```python
from build123d import *

# Parameters (mm, degrees)
SKETCH_2_W                       = 41
SKETCH_2_H                       = 41
EXTRUDE_1_DEPTH                  = 14.3
EXTRUDE_2_DEPTH                  = 1
SKETCH_4_R                       = 7.75
EXTRUDE_3_DEPTH                  = 8
SKETCH_5_R                       = 5.5
EXTRUDE_4_DEPTH                  = 2
SKETCH_6_R                       = 7
EXTRUDE_5_DEPTH                  = 5.2
FILLET_1_R                       = 1
EXTRUDE_6_DEPTH                  = 0.4
SKETCH_11_W                      = 11.5
SKETCH_11_H                      = 6
CUT_EXTRUDE_1_DEPTH              = 7
SKETCH_12_W                      = 11
SKETCH_12_H                      = 4.8
EXTRUDE_7_DEPTH                  = 8.5
SKETCH_13_R                      = 0.5
EXTRUDE_8_DEPTH                  = 3
SKETCH_14_R                      = 1
EXTRUDE_9_DEPTH                  = 2
EXTRUDE_9_DIRECTION_2_REACH      = 48.597
EXTRUDE_9_DIRECTION_2_END_RADIUS = 7.75
SKETCH_15_R                      = 1.5
EXTRUDE_10_DEPTH                 = 1.5


with BuildPart() as part:
    # 草图2 → 凸台-拉伸1 (new body)
    with BuildSketch(Plane.XY):
        Rectangle(SKETCH_2_W, SKETCH_2_H)
    extrude(amount=EXTRUDE_1_DEPTH)

    # 草图3 → 凸台-拉伸2 (add)
    with BuildSketch(Plane.XY.offset(14.3)):
        with BuildLine():
            Line((-11.808683246, 15.061374439), (-6.531779188, 9.784470381))
            ThreePointArc((-6.531779188, 9.784470381), (-5.963517237, 9.501263014), (-5.339283039, 9.617279066))
            ThreePointArc((-5.339283039, 9.617279066), (0, 11), (5.339283039, 9.617279066))
            ThreePointArc((5.339283039, 9.617279066), (5.963517237, 9.501263014), (6.531779188, 9.784470381))
            Line((6.531779188, 9.784470381), (11.808683246, 15.061374439))
            ThreePointArc((11.808683246, 15.061374439), (15.061374439, 15.061374439), (15.061374439, 11.808683246))
            Line((15.061374439, 11.808683246), (9.784470381, 6.531779188))
            ThreePointArc((9.784470381, 6.531779188), (9.501263014, 5.963517237), (9.617279066, 5.339283039))
            ThreePointArc((9.617279066, 5.339283039), (11, 0), (9.617279066, -5.339283039))
            ThreePointArc((9.617279066, -5.339283039), (9.501263014, -5.963517237), (9.784470381, -6.531779188))
            Line((9.784470381, -6.531779188), (15.061374439, -11.808683246))
            ThreePointArc((15.061374439, -11.808683246), (15.061374439, -15.061374439), (11.808683246, -15.061374439))
            Line((11.808683246, -15.061374439), (6.531779188, -9.784470381))
            ThreePointArc((6.531779188, -9.784470381), (5.963517237, -9.501263014), (5.339283039, -9.617279066))
            ThreePointArc((5.339283039, -9.617279066), (0, -11), (-5.339283039, -9.617279066))
            ThreePointArc((-5.339283039, -9.617279066), (-5.963517237, -9.501263014), (-6.531779188, -9.784470381))
            Line((-6.531779188, -9.784470381), (-11.808683246, -15.061374439))
            ThreePointArc((-11.808683246, -15.061374439), (-15.061374439, -15.061374439), (-15.061374439, -11.808683246))
            Line((-15.061374439, -11.808683246), (-9.784470381, -6.531779188))
            ThreePointArc((-9.784470381, -6.531779188), (-9.501263014, -5.963517237), (-9.617279066, -5.339283039))
            ThreePointArc((-9.617279066, -5.339283039), (-11, 0), (-9.617279066, 5.339283039))
            ThreePointArc((-9.617279066, 5.339283039), (-9.501263014, 5.963517237), (-9.784470381, 6.531779188))
            Line((-9.784470381, 6.531779188), (-15.061374439, 11.808683246))
            ThreePointArc((-15.061374439, 11.808683246), (-15.061374439, 15.061374439), (-11.808683246, 15.061374439))
        make_face()
    extrude(amount=EXTRUDE_2_DEPTH)

    # 草图4 → 凸台-拉伸3 (add)
    with BuildSketch(Plane.XY.offset(15.3)):
        Circle(SKETCH_4_R)
    extrude(amount=EXTRUDE_3_DEPTH)

    # 草图5 → 凸台-拉伸4 (add)
    with BuildSketch(Plane.XY.offset(23.3)):
        Circle(SKETCH_5_R)
    extrude(amount=EXTRUDE_4_DEPTH)

    # 草图6 → 凸台-拉伸5 (add)
    with BuildSketch(Plane.XY.offset(25.3)):
        Circle(SKETCH_6_R)
    extrude(amount=EXTRUDE_5_DEPTH)

    # 草图7 → 切除-旋转3 (revolve, cut)
    with BuildSketch(Plane(origin=(0, 0, 0), x_dir=(1, 0, 0), z_dir=(0, 1, 0)), mode=Mode.PRIVATE) as cut_revolve_3_sk:
        with BuildLine():
            Line((-6.8, -30.5), (-5.688128428, -28.574181946))
            ThreePointArc((-5.688128428, -28.574181946), (-4.965242644, -28.084479441), (-4.133231164, -28.349298811))
            ThreePointArc((-4.133231164, -28.349298811), (-2.225332237, -29.572063929), (0, -30))
            Line((0, -30), (0, -30.5))
            Line((0, -30.5), (-6.8, -30.5))
        make_face()
    revolve(cut_revolve_3_sk.sketch.rotate(Axis((0, 0, 30.5), (0, 0, -1)), 180), axis=Axis((0, 0, 30.5), (0, 0, -1)), mode=Mode.SUBTRACT)

    # 圆角1
    fillet_1_edges = [part.edges().sort_by_distance(p)[0] for p in [
        (-20.5, 0, 14.3),
        (0, -20.5, 14.3),
        (20.5, 0, 14.3),
        (0, 20.5, 14.3),
        (20.5, -20.5, 7.15),
        (-20.5, -20.5, 7.15),
        (-20.5, 20.5, 7.15),
        (20.5, 20.5, 7.15),
    ]]
    fillet(fillet_1_edges, radius=FILLET_1_R)

    # 草图8 → 凸台-拉伸6 (add)
    with BuildSketch(Plane(origin=(20.5, 0, 0), x_dir=(0, 0, -1), z_dir=(1, 0, 0))):
        with BuildLine():
            Line((-8.887238775, 1.998096443), (0, 2.386121668))
            Line((0, 2.386121668), (0, -2.386121668))
            Line((0, -2.386121668), (-8.887238775, -1.998096443))
            ThreePointArc((-8.887238775, -1.998096443), (-10.8, 0), (-8.887238775, 1.998096443))
        make_face()
    extrude_6 = extrude(amount=EXTRUDE_6_DEPTH)

    # 草图10 → M2 螺纹孔1 (revolve, cut)
    with BuildSketch(Plane(origin=(20.9, 0, 8.8), x_dir=(0, 0, -1), z_dir=(0, 1, 0))):
        Polygon((0, 0), (0, 5.680688495), (0.8, 5.2), (0.8, 0), align=None)
    hole_wizard_m2_1 = revolve(axis=Axis((27.25, 0, 8.8), (-1, 0, 0)), mode=Mode.SUBTRACT)

    # 镜向1: 凸台-拉伸6, M2 螺纹孔1 across plane
    add(extrude_6.mirror(Plane(origin=(0, 0, 0), x_dir=(0, 0, 1), z_dir=(1, 0, 0))))
    add(hole_wizard_m2_1.mirror(Plane(origin=(0, 0, 0), x_dir=(0, 0, 1), z_dir=(1, 0, 0))), mode=Mode.SUBTRACT)

    # 草图11 → 切除-拉伸1 (cut)
    with BuildSketch(Plane(origin=(0, 0, 0), x_dir=(-1, 0, 0), z_dir=(0, 0, -1))):
        with Locations((-4.75, -14)):
            Rectangle(SKETCH_11_W, SKETCH_11_H)
    extrude(amount=-CUT_EXTRUDE_1_DEPTH, mode=Mode.SUBTRACT)

    # 草图12 → 凸台-拉伸7 (add)
    with BuildSketch(Plane(origin=(0, 0, 7), x_dir=(-1, 0, 0), z_dir=(0, 0, -1))):
        with Locations((-4.75, -13.6)):
            Rectangle(SKETCH_12_W, SKETCH_12_H)
    extrude(amount=EXTRUDE_7_DEPTH)

    # 草图13 → 凸台-拉伸8 (add)
    with BuildSketch(Plane(origin=(0, 0, -1.5), x_dir=(-1, 0, 0), z_dir=(0, 0, -1))):
        with Locations((-8.56, -14)):
            Circle(SKETCH_13_R)
        with Locations((-6.02, -14)):
            Circle(SKETCH_13_R)
        with Locations((-3.48, -14)):
            Circle(SKETCH_13_R)
        with Locations((-0.94, -14)):
            Circle(SKETCH_13_R)
    extrude(amount=EXTRUDE_8_DEPTH)

    # 草图14 → 凸台-拉伸9 (add)
    with BuildSketch(Plane(origin=(7.75, 0, 0), x_dir=(0, 0, -1), z_dir=(1, 0, 0))):
        with Locations((-20.3, 0)):
            Circle(SKETCH_14_R)
    extrude(amount=EXTRUDE_9_DEPTH)

    # 凸台-拉伸9 direction 2: up to this cylinder (the profile starts outside it)
    extrude_9_direction_2_end = Plane(origin=(0, 0, 20.3), z_dir=(0, 0, -1)) * Cylinder(EXTRUDE_9_DIRECTION_2_END_RADIUS, 113.694, mode=Mode.PRIVATE)
    # 草图14 → 凸台-拉伸9 direction 2 (add, up to the surface)
    with BuildSketch(Plane(origin=(7.75, 0, 0), x_dir=(0, 0, -1), z_dir=(1, 0, 0)), mode=Mode.PRIVATE) as extrude_9_direction_2_sk1:
        with Locations((-20.3, 0)):
            Circle(SKETCH_14_R)
    extrude_9_direction_2_tool1 = extrude(extrude_9_direction_2_sk1.sketch, amount=-EXTRUDE_9_DIRECTION_2_REACH, mode=Mode.PRIVATE) - extrude_9_direction_2_end
    add(extrude_9_direction_2_tool1.solids().sort_by_distance((7.75, 0, 20.3))[0])
    add(extrude_9_direction_2_tool1.solids().sort_by_distance((7.75, 0, 20.3))[1])

    # 草图15 → 凸台-拉伸10 (add)
    with BuildSketch(Plane(origin=(9.75, 0, 0), x_dir=(0, 0, -1), z_dir=(1, 0, 0))):
        with Locations((-20.3, 0)):
            Circle(SKETCH_15_R)
    extrude(amount=EXTRUDE_10_DEPTH)


solid = part.part
```
Work out the finished part from the listing and answer in its coordinate system (mm). A direction names the side the tool comes from. Round coordinates to 2 decimals unless told otherwise and drop trailing zeros. Write each loop counter-clockwise with the first axis right and the second up, starting at its lowest first coordinate (ties: lowest second). Pieces come first, ordered by that corner, then holes.
1) A cutting plane is placed at A-A on z = 4.5. Determine the outline of the cut face in (x, y).
2) Consider probe 1 along Y at (x, z) = (4, 2); probe 2 along Y at (x, z) = (16.8, 8.8); probe 3 along Z at (x, y) = (-9.5, -16.5). Determine where each line is inside the solid, lowest interval first.
3) Flat-ended cylindrical pins translate along their axes: P1, Ø6, axis at y = -6, z = 14.5, coming from the +X side; P2, Ø12, axis at x = -6.5, y = 4.5, coming from the -Z side; P3, Ø1.5, axis at x = 5.5, z = 21.5, coming from the -Y side. Find the tip coordinate at first contact, or state that the pin passes through.
4) A cutting plane is placed at B-B on z = 20.3. Determine the outline of the cut face in (x, y).
5) Which of the six approach directions +Z, -Z, +X, -X, +Y, -Y give full straight-line access (tool end or side, diameter ignored) to faces 5 (the face through (-11, 0, 15)), 6 (the face through (-0.75, -14, 3)), 7 (the face through (-15.097, 15.025, 14.793)), 8 (the face through (15.303, -0.006, 8.939)), 9 (the face through (8.7, 0, 21.3))?
6) Determine the mould class of faces 1 (the face through (11.25, 0, 20)), 2 (the face through (-20.5, 0, 11)), 3 (the face through (-1.19, -5.37, 24.29)), 4 (the face through (0, 11, 15)) for opening direction X: pulls with the +X half, pulls with the -X half, needs draft (parallel to the pull), parting line crosses it, or undercut.
Entries:
1. outline: (-20.9, -2.19) - (-20.5, -2.19) - (-20.5, -19.5) arc R1 ccw to (-19.5, -20.5) - (19.5, -20.5) arc R1 ccw to (20.5, -19.5) - (20.5, -2.19) - (20.9, -2.19) - (20.9, 2.19) - (20.5, 2.19) - (20.5, 19.5) arc R1 ccw to (19.5, 20.5) - (-19.5, 20.5) arc R1 ccw to (-20.5, 19.5) - (-20.5, 2.19) - (-20.9, 2.19) - close; (-0.75, -16) - (10.25, -16) - (10.25, -11.2) - (-0.75, -11.2) - close; hole (-1, -17) - (10.5, -17) - (10.5, -11) - (-1, -11) - close
2. probe 1: y = -20.5 to -17, -16 to -11.2, -11 to 20.5
2. probe 2: y = -20.5 to -0.8, 0.8 to 20.5
2. probe 3: z = 0 to 14.3
3. P1: stops at x = 20.5
3. P2: stops at z = 0
3. P3: stops at y = -6.12
4. outline: (7.69, -1) - (9.75, -1) - (9.75, -1.5) - (11.25, -1.5) - (11.25, 1.5) - (9.75, 1.5) - (9.75, 1) - (7.69, 1) arc R7.75 ccw (long way) to start
5. face 5: +Z, -X
5. face 6: -Z
5. face 7: +Z
5. face 8: +X
5. face 9: none
6. face 1: pulls with the +X half
6. face 2: pulls with the -X half
6. face 3: parting line crosses it
6. face 4: undercut
